Verification items for the finished model (mm, model axes). Face numbers are marked on the shaded views. A direction names the side the tool comes from. Coordinates: 2 decimals unless noted, no trailing zeros. Order: outer loops, then holes, each group sorted by start corner. A loop starts at its lowest first (then second) coordinate and runs counter-clockwise, first axis right, second up.
Q1. Cross-section at C-C, the plane z = 13.5. Record the boundary of the cut face in (x, y), and give its area (3 significant figures).
Q2. Set-up check for the marked faces 4, 5 and 6: record each of +Z, -Z, +X, -X, +Y, -Y from which the full face is reachable in a straight line by a thin tool's end or side.
Q3. Cross-section at A-A, the plane x = 0. Count the separate pieces of the cut face and the enclosed holes in it, and give its area (3 significant figures).
Q4. Draft check along X on the marked faces 1, 2 and 3. Enter one of: pulls with the +X half, pulls with the -X half, needs draft (parallel to the pull), parting line crosses it, or undercut.
Q5. Thickness scan on line 1 (Y direction, x = 0, z = 1.65); line 2 (Y direction, x = 0, z = 7.75); line 3 (Z direction, x = 1.25, y = -62). Record the ranges inside material, lowest first.
Q6. Cross-section at B-B, the plane y = -91. Record the boundary of the cut face in (x, z), and give its area (3 significant figures).
Q7. Depth check by flat-ended pin: P1, Ø0.8, axis at x = 0.5, z = 4.5, coming from the -Y side; P2, Ø4, axis at y = -6, z = 14, coming from the +X side; P3, Ø4, axis at y = -64.5, z = 3.5, coming from the -X side; P4, Ø2.5, axis at y = -44, z = 3.5, coming from the +X side. Enter the tip coordinate at first touch or a pass-through.
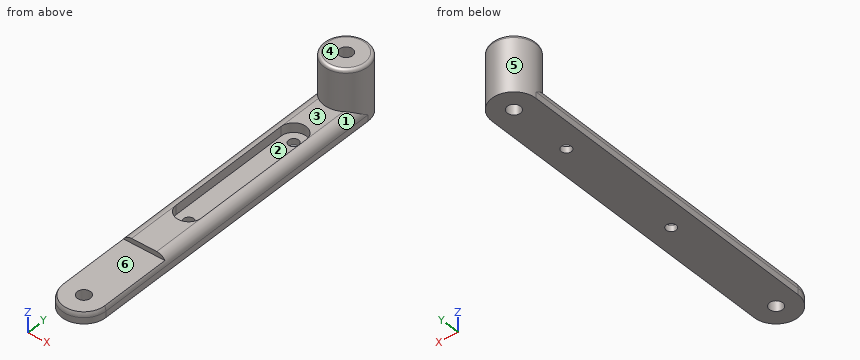
from build123d import *

# Parameters (mm, degrees)
SKETCH1_R           = 7
BOSS_EXTRUDE1_DEPTH = 18
SKETCH2_W           = 14
SKETCH2_H           = 100
BOSS_EXTRUDE2_DEPTH = 5
SKETCH8_R           = 2.1
CUT_EXTRUDE5_DEPTH  = 18
SKETCH9_R           = 7
BOSS_EXTRUDE4_DEPTH = 5
FILLET3_R           = 3
CUT_EXTRUDE6_DEPTH  = 3
SKETCH10_R          = 1.6
CUT_EXTRUDE7_DEPTH  = 3
SKETCH11_W          = 14
SKETCH11_H          = 30
CUT_EXTRUDE8_DEPTH  = 1.5
SKETCH12_R          = 2.1
CUT_EXTRUDE9_DEPTH  = 4
FILLET4_R           = 1


with BuildPart() as part:
    # Sketch1 → Boss-Extrude1 (new body)
    with BuildSketch(Plane.XY):
        Circle(SKETCH1_R)
    extrude(amount=BOSS_EXTRUDE1_DEPTH)

    # Sketch2 → Boss-Extrude2 (add)
    with BuildSketch(Plane.XY):
        with Locations((0, -50)):
            Rectangle(SKETCH2_W, SKETCH2_H)
    extrude(amount=BOSS_EXTRUDE2_DEPTH)

    # Sketch8 → Cut-Extrude5 (cut)
    with BuildSketch(Plane.XY.offset(18)):
        Circle(SKETCH8_R)
    extrude(amount=-CUT_EXTRUDE5_DEPTH, mode=Mode.SUBTRACT)

    # Sketch9 → Boss-Extrude4 (add)
    with BuildSketch(Plane.XY.offset(5)):
        with Locations((0, -100)):
            Circle(SKETCH9_R)
    extrude(amount=-BOSS_EXTRUDE4_DEPTH)

    # Fillet3
    # the kernel refuses this fillet: 3 mm, written as the material it takes off along each edge
    with BuildSketch(Plane(origin=(7, 7.5, 5), x_dir=(-1, 0, 0), z_dir=(0, -1, 0))) as fillet3_piece_1_section:
        with BuildLine():
            CenterArc((FILLET3_R, FILLET3_R), FILLET3_R, 180, 90)
            Line((0, FILLET3_R), (0, 0))
            Line((0, 0), (FILLET3_R, 0))
        make_face()
    fillet3_piece_1 = extrude(amount=107.5, mode=Mode.PRIVATE)
    fillet3_piece_1 = fillet3_piece_1 - Plane(origin=(0, 0, 4.308954976), x_dir=(1, 0, 0), z_dir=(0, 0, -1)) * Cylinder(7, 227, mode=Mode.PRIVATE)
    add(fillet3_piece_1, mode=Mode.SUBTRACT)
    with BuildSketch(Plane(origin=(0, -100, 5), x_dir=(-1, 0, 0), z_dir=(0, 1, 0))) as fillet3_piece_2:
        with BuildLine():
            CenterArc((7 - FILLET3_R, -FILLET3_R), FILLET3_R, 0, 90)
            Line((7, -FILLET3_R), (7, 0))
            Line((7, 0), (7 - FILLET3_R, 0))
        make_face()
    revolve(axis=Axis((0, -100, 5), (0, 0, 1)), revolution_arc=180, mode=Mode.SUBTRACT)
    with BuildSketch(Plane(origin=(-7, -100, 5), x_dir=(0, 0, -1), z_dir=(0, 1, 0))) as fillet3_piece_3_section:
        with BuildLine():
            CenterArc((FILLET3_R, -FILLET3_R), FILLET3_R, 90, 90)
            Line((0, -FILLET3_R), (0, 0))
            Line((0, 0), (FILLET3_R, 0))
        make_face()
    fillet3_piece_3 = extrude(amount=107.5, mode=Mode.PRIVATE)
    fillet3_piece_3 = fillet3_piece_3 - Plane(origin=(0, 0, 4.308954508), x_dir=(1, 0, 0), z_dir=(0, 0, -1)) * Cylinder(7, 227, mode=Mode.PRIVATE)
    add(fillet3_piece_3, mode=Mode.SUBTRACT)

    # Sketch6 → Cut-Extrude6 (cut)
    with BuildSketch(Plane.XY.offset(5)):
        with BuildLine():
            Line((4, -20), (4, -60))
            ThreePointArc((4, -60), (0, -64), (-4, -60))
            Line((-4, -60), (-4, -20))
            ThreePointArc((-4, -20), (0, -16), (4, -20))
        make_face()
    extrude(amount=-CUT_EXTRUDE6_DEPTH, mode=Mode.SUBTRACT)

    # Sketch10 → Cut-Extrude7 (cut)
    with BuildSketch(Plane.XY.offset(2)):
        with Locations((0, -20)):
            Circle(SKETCH10_R)
        with Locations((0, -60)):
            Circle(SKETCH10_R)
    extrude(amount=-CUT_EXTRUDE7_DEPTH, mode=Mode.SUBTRACT)

    # Sketch11 → Cut-Extrude8 (cut)
    with BuildSketch(Plane.XY.offset(5)):
        with Locations((0, -92)):
            Rectangle(SKETCH11_W, SKETCH11_H)
    extrude(amount=-CUT_EXTRUDE8_DEPTH, mode=Mode.SUBTRACT)

    # Sketch12 → Cut-Extrude9 (cut)
    with BuildSketch(Plane.XY.offset(3.5)):
        with Locations((0, -100)):
            Circle(SKETCH12_R)
    extrude(amount=-CUT_EXTRUDE9_DEPTH, mode=Mode.SUBTRACT)

    # Fillet4
    fillet4_edges = [part.edges().sort_by_distance(p)[0] for p in [
        (-7, 0, 18),
    ]]
    fillet(fillet4_edges, radius=FILLET4_R)


solid = part.part
Check values:
1. outline: circle Ø14 at (0, 0); hole circle Ø4.2 at (0, 0)
1. area: 140 mm2
2. face 4: +Z, +X, -X, +Y, -Y
2. face 5: +Z
2. face 6: +Z, +X, -X, -Y
3. separate pieces: 5
3. enclosed holes: 0
3. area: 459 mm2
4. face 1: pulls with the +X half
4. face 2: undercut
4. face 3: needs draft
5. line 1: y = -107 to -102.1, -97.9 to -61.6, -58.4 to -21.6, -18.4 to -2.1, 2.1 to 7
5. line 2: y = -7 to -2.1, 2.1 to 7
5. line 3: z = 0 to 2
6. outline: (-7, 0) - (7, 0) - (7, 2) arc R3 ccw to (6.6, 3.5) - (-6.6, 3.5) arc R3 ccw to (-7, 2) - close
6. area: 48.6 mm2
7. P1: stops at y = -77
7. P2: stops at x = 5.74
7. P3: stops at x = -7
7. P4: stops at x = 6.99
